The drawing under review shows one solid part. Ordinate dimensions are in mm from its lowest x, y, z. Coordinates: 2 decimals unless noted, no trailing zeros. Loops run counter-clockwise (first coordinate to the right, second up) from the corner with the lowest first, then second, coordinate; pieces in that order, holes last. Notation, with made-up numbers: (-10.5, 43.25) - (-4.5, 43.25) arc R19 cw to (-4.5, 70.25) - close; hole circle Ø9 at (73.25, -20.75). An arc over 180 degrees is marked (long way). Use one line per item in the form item = value. Start each with the question number.
1. Add section B-B on y = 11. Give the boundary of the cut face in (x, z), and give its area (3 significant figures).
2. Add section C-C on x = 17.5. Give the boundary of the cut face in (y, z).
3. To check wall thickness, follow probe 1 along Z at (x, y) = (26.5, 15.5); probe 2 along Z at (x, y) = (2.5, 8.5) (1 decimal); probe 3 along Y at (x, z) = (8, 15) (1 decimal). State the ranges of each line that lie inside material, in increasing order.
4. For pin 1 Ø1 at (y, z) = (31, 69.5) entering from +X (1 decimal); pin 2 Ø1 at (x, z) = (14.5, 53) entering from +Y; pin 3 Ø6 at (y, z) = (11, 15) entering from +X, all flat-tipped, find the tip position at first contact; note any pin that passes through.
5. Add section D-D on z = 46. Give the boundary of the cut face in (x, y), and give its area (3 significant figures).
6. Add section A-A on z = 15. Give the boundary of the cut face in (x, y).
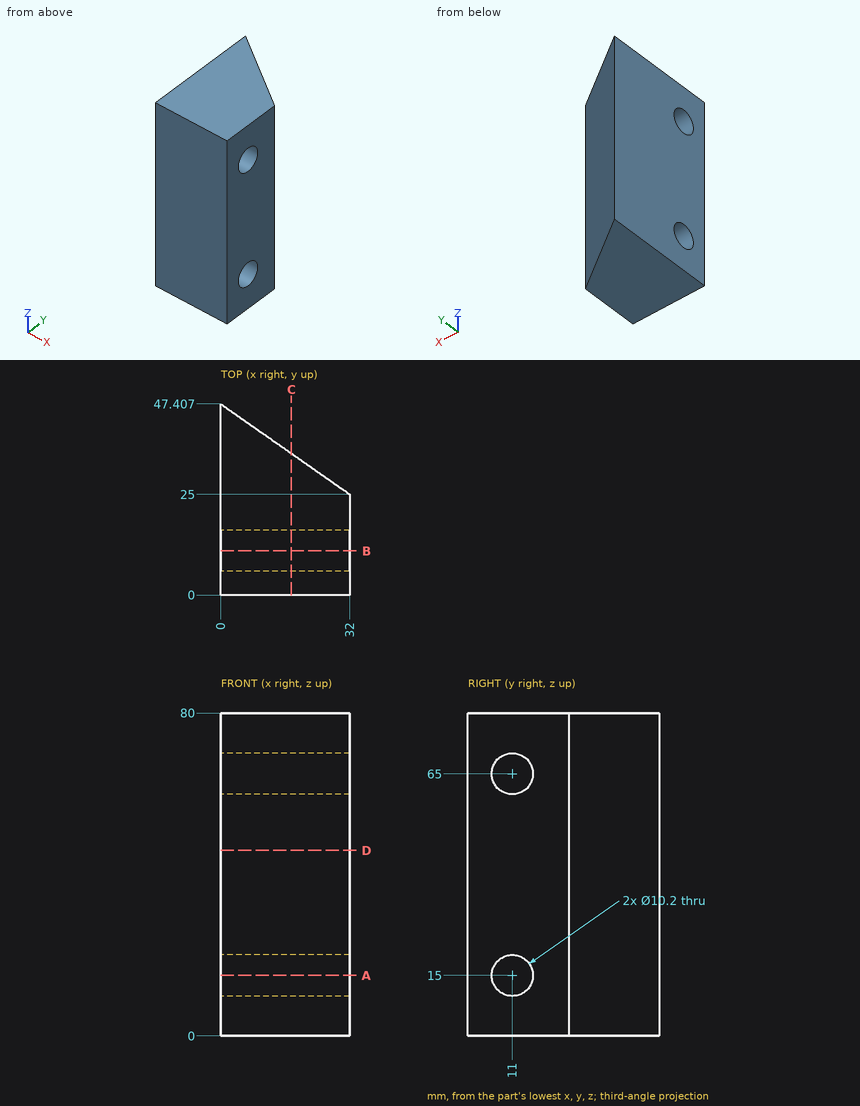
Conclusion:
q1.outline = (0, 0) - (32, 0) - (32, 9.9) - (0, 9.9) - close; (0, 20.1) - (32, 20.1) - (32, 59.9) - (0, 59.9) - close; (0, 70.1) - (32, 70.1) - (32, 80) - (0, 80) - close
q1.area = 1,910 mm^2
q2.outline = (0, 0) - (35.15, 0) - (35.15, 80) - (0, 80) - close; hole circle Ø10.2 at (11, 15); hole circle Ø10.2 at (11, 65)
q3.probe_1 = 0 to 12.6, 17.4 to 62.6, 67.4 to 80
q3.probe_2 = 0 to 10.6, 19.4 to 60.6, 69.4 to 80
q3.probe_3 = 0 to 5.9, 16.1 to 41.8
q4.pin_1 = 24.1
q4.pin_2 = 37.6
q4.pin_3 = through
q5.outline = (0, 0) - (32, 0) - (32, 25) - (0, 47.41) - close
q5.area = 1,160 mm^2
q6.outline = (0, 0) - (32, 0) - (32, 5.9) - (0, 5.9) - close; (0, 16.1) - (32, 16.1) - (32, 25) - (0, 47.41) - close
